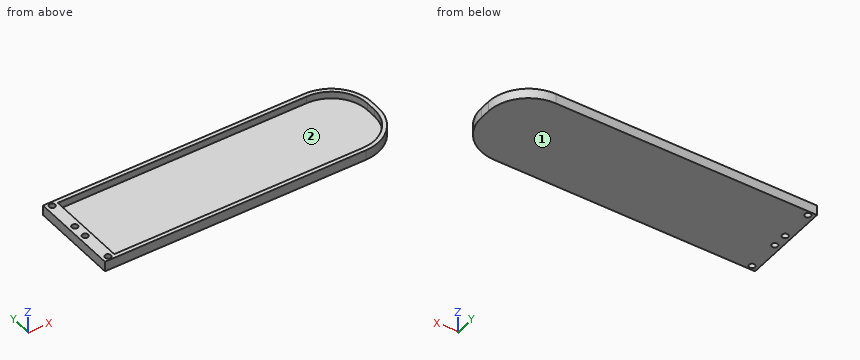
from build123d import *

# Parameters (mm, degrees)
BOSS_EXTRUDE1_DEPTH = 3
SKETCH1_3_R         = 3
BOSS_EXTRUDE2_DEPTH = 10


with BuildPart() as part:
    # Sketch1 → Boss-Extrude1 (new body)
    with BuildSketch(Plane.XY):
        with BuildLine():
            Line((-138, -45), (110, -45))
            ThreePointArc((110, -45), (138.284271247, -33.284271247), (150, -5))
            Line((150, -5), (150, 5))
            ThreePointArc((150, 5), (138.284271247, 33.284271247), (110, 45))
            Line((110, 45), (-138, 45))
            Line((-138, 45), (-138, -45))
        make_face()
    extrude(amount=BOSS_EXTRUDE1_DEPTH)

    # Sketch1_3 → Boss-Extrude2 (add)
    with BuildSketch(Plane.XY):
        Polygon((-150, -45), (-138, -45), (-138, -41), (-138, 41), (-138, 45), (-150, 45), align=None)
        with Locations((-144, -40.5)):
            Circle(SKETCH1_3_R, mode=Mode.SUBTRACT)
        with Locations((-144, -7.5)):
            Circle(SKETCH1_3_R, mode=Mode.SUBTRACT)
        with Locations((-144, 7.5)):
            Circle(SKETCH1_3_R, mode=Mode.SUBTRACT)
        with Locations((-144, 40.5)):
            Circle(SKETCH1_3_R, mode=Mode.SUBTRACT)
        with BuildLine():
            Line((-138, -45), (110, -45))
            ThreePointArc((110, -45), (138.284271247, -33.284271247), (150, -5))
            Line((150, -5), (150, 5))
            ThreePointArc((150, 5), (138.284271247, 33.284271247), (110, 45))
            Line((110, 45), (-138, 45))
            Line((-138, 45), (-138, 41))
            Line((-138, 41), (110, 41))
            ThreePointArc((110, 41), (135.455844123, 30.455844123), (146, 5))
            Line((146, 5), (146, -5))
            ThreePointArc((146, -5), (135.455844123, -30.455844123), (110, -41))
            Line((110, -41), (-138, -41))
            Line((-138, -41), (-138, -45))
        make_face()
    extrude(amount=BOSS_EXTRUDE2_DEPTH)


solid = part.part
Source: CAD feature listing. Evaluate the final solid. Frame: model axes, mm. Face numbers are marked on the shaded views. Give positions to 0.01 mm unless a question says otherwise; leave off trailing zeros. Write each loop counter-clockwise with the first axis right and the second up, starting at its lowest first coordinate (ties: lowest second). Pieces come first, ordered by that corner, then holes. Notation, with made-up numbers: (-22.75, -20.75) -> (18.25, -20.75) arc R11 ccw to (18.25, -9.75) -> close; hole circle Ø9 at (-35.75, 13.5). An arc over 180 degrees is marked (long way). Return JSON: item names as keys, results as strings. Group by question number.
1. Section D-D, the plane x = -74. Output: boundary loops of the cut face in (y, z), then the cut area to 3 significant figures.
2. Mould query, pull axis X, two halves, no side actions, for the marked faces 1 and 2. Classes: +X half, -X half, draft (parallel to the pull), parting line (faces both ways), or undercut.
3. Pin query (flat end, axial travel): pin 1 Ø8 at (x, y) = (38.5, -27.5) entering from +Z; pin 2 Ø5 at (y, z) = (33, 7.5) entering from +X. Return the tip coordinate at first contact, or that it passes through.
4. Section B-B, the plane z = 6.75. Output: boundary loops of the cut face in (x, y), then the cut area to 3 significant figures.
5. Section A-A, the plane x = -144. Output: boundary loops of the cut face in (y, z), then the cut area to 3 significant figures.
6. Section C-C, the plane y = -1. Output: boundary loops of the cut face in (x, z), then the cut area to 3 significant figures.
7. Material intervals for line 1 (Y direction, x = -144, z = 5.5); line 2 (Y direction, x = -25, z = 5.75); line 3 (X direction, y = -7, z = 7.75), sorted ascending. Write a range as from..to.
Determined:
{
 "1": {"outline": "(-45, 0) -> (45, 0) -> (45, 10) -> (41, 10) -> (41, 3) -> (-41, 3) -> (-41, 10) -> (-45, 10) -> close", "area": "326 mm2"},
 "2": {"face 1": "draft", "face 2": "undercut"},
 "3": {"pin 1": "stops at z = 3", "pin 2": "stops at x = 140.82"},
 "4": {"outline": "(-150, -45) -> (110, -45) arc R40 ccw to (150, -5) -> (150, 5) arc R40 ccw to (110, 45) -> (-150, 45) -> close; hole circle Ø6 at (-144, -40.5); hole circle Ø6 at (-144, -7.5); hole circle Ø6 at (-144, 7.5); hole circle Ø6 at (-144, 40.5); hole (-138, -41) -> (110, -41) arc R36 ccw to (146, -5) -> (146, 5) arc R36 ccw to (110, 41) -> (-138, 41) -> close", "area": "3,470 mm2"},
 "5": {"outline": "(-45, 0) -> (-43.5, 0) -> (-43.5, 10) -> (-45, 10) -> close; (-37.5, 0) -> (-10.5, 0) -> (-10.5, 10) -> (-37.5, 10) -> close; (-4.5, 0) -> (4.5, 0) -> (4.5, 10) -> (-4.5, 10) -> close; (10.5, 0) -> (37.5, 0) -> (37.5, 10) -> (10.5, 10) -> close; (43.5, 0) -> (45, 0) -> (45, 10) -> (43.5, 10) -> close", "area": "660 mm2"},
 "6": {"outline": "(-150, 0) -> (150, 0) -> (150, 10) -> (146, 10) -> (146, 3) -> (-138, 3) -> (-138, 10) -> (-150, 10) -> close", "area": "1,010 mm2"},
 "7": {"line 1": "y = -45..-43.5, -37.5..-10.5, -4.5..4.5, 10.5..37.5, 43.5..45", "line 2": "y = -45..-41, 41..45", "line 3": "x = -150..-146.96, -141.04..-138, 145.94..149.95"}
}
